Check sheet for the modelled part. Datum: model origin and axes. Units: mm. Give positions to 0.01 mm unless a question says otherwise; leave off trailing zeros. Write each loop counter-clockwise with the first axis right and the second up, starting at its lowest first coordinate (ties: lowest second). Pieces come first, ordered by that corner, then holes. Notation, with made-up numbers: (56, -16) -> (107, -16) arc R7 cw to (107, -7) -> close; hole circle Ø8 at (56, 54). An arc over 180 degrees is marked (long way). Write each question's results on one line, items separated by ' | '. Start each with the question number.
```python
from build123d import *

# Parameters (mm, degrees)
BASE_FLANGE1_DEPTH = 1.89738
SKETCH6_R          = 2.5
CUT_EXTRUDE1_DEPTH = 1.89738
SKETCH7_W          = 5
SKETCH7_H          = 15
CUT_EXTRUDE2_DEPTH = 10


# Sheet-metal steps are written as plain solids
with BuildPart() as part:
    # Sketch1 → Base-Flange1 (new body)
    with BuildSketch(Plane(origin=(0, 0, 0), x_dir=(1, 0, 0), z_dir=(0, 1, 0))):
        Polygon((43.041223022, 34.251798561), (48.041223022, 34.251798561), (48.041223022, 24.251798561), (43.041223022, 24.251798561), (43.041223022, -147.248201439), (-111.528776978, -147.248201439), (-111.528776978, 24.251798561), (-116.528776978, 24.251798561), (-116.528776978, 34.251798561), (-111.528776978, 34.251798561), (-111.528776978, 52.751798561), (43.041223022, 52.751798561), align=None)
    extrude(amount=-BASE_FLANGE1_DEPTH)

    # Sketch6 → Cut-Extrude1 (cut)
    with BuildSketch(Plane.XZ.offset(1.89738)):
        with Locations(Location((-107.528776978, 122.248201439, 0), (0, 0, 270))):
            Circle(SKETCH6_R)
        with Locations(Location((39.041223022, 142.248201439, 0), (0, 0, 270))):
            Circle(SKETCH6_R)
        with Locations(Location((-110.028776978, -29.729970338, 0), (0, 0, 270))):
            Circle(SKETCH6_R)
        with Locations(Location((41.503528065, -30.503445529, 0), (0, 0, 270))):
            Circle(SKETCH6_R)
    extrude(amount=-CUT_EXTRUDE1_DEPTH, mode=Mode.SUBTRACT)

    # Sketch7 → Cut-Extrude2 (cut)
    with BuildSketch(Plane(origin=(0, 0, 0), x_dir=(1, 0, 0), z_dir=(0, 1, 0))):
        with Locations((-109.028776978, -139.748201439)):
            Rectangle(SKETCH7_W, SKETCH7_H)
    extrude(amount=-CUT_EXTRUDE2_DEPTH, mode=Mode.SUBTRACT)


solid = part.part
```
Item 1: Section check B-B on z = 92. Record the boundary of the cut face in (x, y), then the cut area to 3 significant figures.
Item 2: Thickness scan on probe 1 along X at (y, z) = (-1.35, -30.5); probe 2 along X at (y, z) = (-0.35, 135); probe 3 along X at (y, z) = (-0.6, 11.5). Record the ranges inside material, lowest first. Write a range as from..to.
Item 3: Depth check by flat-ended pin: pin 1 Ø0.6 at (y, z) = (-1, 139) entering from -X; pin 2 Ø0.6 at (x, y) = (-114, -1) entering from +Z; pin 3 Ø0.9 at (y, z) = (-0.5, 17) entering from -X. Enter the tip coordinate at first touch or a pass-through.
Item 4: Section check A-A on y = -1.2. Record the boundary of the cut face in (x, z).
Item 5: Mould release check, pull along Z, two halves, no side actions. Record for faces 1 (the cylindrical face through (-107.55, -0.96, -29.4)), 2 (the flat face through (-33, -1.897, 46)): pulls with the +Z half, pulls with the -Z half, needs draft (parallel to the pull), parting line crosses it, or undercut.
Check sheet entries:
1) outline: (-111.53, -1.9) -> (43.04, -1.9) -> (43.04, 0) -> (-111.53, 0) -> close | area: 293 mm^2
2) probe 1: x = -116.53..-112.41, -107.65..39, 44..48.04 | probe 2: x = -106.53..43.04 | probe 3: x = -111.53..43.04
3) pin 1: stops at x = -106.53 | pin 2: stops at z = -24.25 | pin 3: stops at x = -111.53
4) outline: (-116.53, -34.25) -> (-111.53, -34.25) -> (-111.53, -52.75) -> (43.04, -52.75) -> (43.04, -34.25) -> (48.04, -34.25) -> (48.04, -24.25) -> (43.04, -24.25) -> (43.04, 147.25) -> (-106.53, 147.25) -> (-106.53, 132.25) -> (-111.53, 132.25) -> (-111.53, -24.25) -> (-116.53, -24.25) -> close; hole circle Ø5 at (-110.03, -29.73); hole circle Ø5 at (-107.53, 122.25); hole circle Ø5 at (39.04, 142.25); hole circle Ø5 at (41.5, -30.5)
5) face 1: undercut | face 2: needs draft
